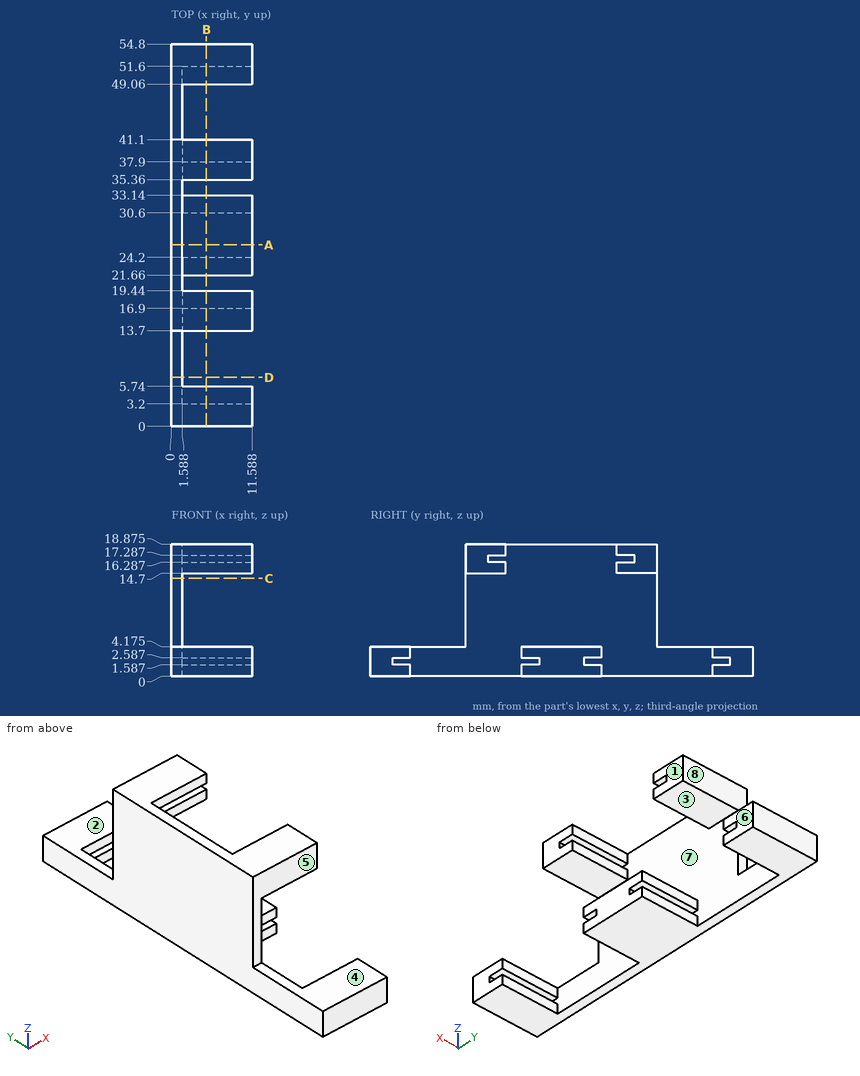
Input: dimensioned drawing with shaded views. Units: mm. Origin: part minimum x, y, z. A direction names the side the tool comes from. Coordinates: 2 decimals unless noted, no trailing zeros. Write each loop counter-clockwise with the first axis right and the second up, starting at its lowest first coordinate (ties: lowest second). Pieces come first, ordered by that corner, then holes. Notation, with made-up numbers: (64.5, 64) -> (68.5, 64) arc R16 ccw to (68.5, 94) -> close; hole circle Ø8 at (68.5, 42.5). An arc over 180 degrees is marked (long way). Return JSON: item names as keys, results as strings. Group by question number.
1) Section query A-A, the plane y = 26. Return loops of the section in (x, z) (1 decimal).
2) Section query D-D, the plane y = 7. Return loops of the section in (x, z) (1 decimal).
3) Section query B-B, the plane x = 5. State how many separate pieces and enclosed holes the cut face has.
4) Mould query, pull axis Y, two halves, no side actions, for the marked faces 5, 6, 7 and 8. Classes: +Y half, -Y half, draft (parallel to the pull), parting line (faces both ways), or undercut.
5) Contact query for flat-ended pins moving along their axis: P1, Ø0.8, axis at x = 6.5, y = 31.5, coming from the +Z side (1 decimal); P2, Ø4, axis at x = 6, z = 14, coming from the +Y side; P3, Ø6.5, axis at x = 6, y = 38, coming from the -Z side. Output: stop coordinate, or through.
6) Set-up query: the marked faces 1, 2, 3 and 4. Return all of +Z, -Z, +X, -X, +Y, -Y with unobstructed straight access to the full face (end or side cutting, diameter ignored); none if empty.
7) Ray query, line 1 along Y through (x, z) = (10.5, 16); line 2 along Z through (x, y) = (4.5, 18) (1 decimal); line 3 along Z through (x, y) = (8.5, 22.5) (1 decimal). Return the intervals inside material, ascending.
8) Section query C-C, the plane z = 14. Return loops of the section in (x, y).
From the geometry:
{
 "1": {"outline": "(0, 0) -> (11.6, 0) -> (11.6, 4.2) -> (1.6, 4.2) -> (1.6, 18.9) -> (0, 18.9) -> close"},
 "2": {"outline": "(0, 0) -> (1.6, 0) -> (1.6, 4.2) -> (0, 4.2) -> close"},
 "3": {"separate pieces": "5", "enclosed holes": "0"},
 "4": {"face 5": "-Y half", "face 6": "draft", "face 7": "undercut", "face 8": "+Y half"},
 "5": {"P1": "z = 4.2", "P2": "y = 41.1", "P3": "z = 14.7"},
 "6": {"face 1": "+Z, -Z, +X, +Y, -Y", "face 2": "+Z, +X, -X, +Y", "face 3": "-Z, +X, +Y, -Y", "face 4": "+Z, +X, -X, -Y"},
 "7": {"line 1": "13.7 to 19.44, 35.36 to 41.1", "line 2": "14.7 to 16.3, 17.3 to 18.9", "line 3": "0 to 1.6, 2.6 to 4.2"},
 "8": {"outline": "(0, 13.7) -> (1.59, 13.7) -> (1.59, 41.1) -> (0, 41.1) -> close"}
}
